Input: part model. Units: mm. Frame: model coordinates. A direction names the side the tool comes from. Give positions to 0.01 mm unless a question says otherwise; leave off trailing zeros. Loops run counter-clockwise (first coordinate to the right, second up) from the corner with the lowest first, then second, coordinate; pieces in that order, holes last. Notation, with made-up numbers: (-15.75, -33.75) - (37.25, -33.75) arc R10 cw to (37.25, -29.75) - close; hole circle Ø6 at (66.5, -18). An arc over 180 degrees is marked (long way). One line per item, written item: value.
from build123d import *

# Parameters (mm, degrees)
BOSS_EXTRUDE1_DEPTH     = 32
SKETCH2_R               = 22.5
BOSS_EXTRUDE4_DEPTH     = 10
CUT_EXTRUDE1_DEPTH      = 80.029560932
CUT_EXTRUDE1_DEPTH_BACK = 80.029560932
SKETCH3_R               = 5
FILLET3_R               = 11
FILLET4_RADIUS          = 16
FILLET4_LENGTH          = 4.5
FILLET5_RADIUS          = 16
FILLET5_LENGTH          = 4.5
CUT_EXTRUDE2_DEPTH      = 74.711106836
CUT_EXTRUDE2_DEPTH_BACK = 74.711106836
SKETCH4_R               = 3


with BuildPart() as part:
    # Sketch1 → Boss-Extrude1 (new body)
    with BuildSketch(Plane.XY):
        Polygon((-19.112903226, 28.185483871), (-19.112903226, -26.814516129), (43.887096774, -26.814516129), (43.887096774, 28.185483871), (39.387096774, 28.185483871), (39.387096774, -16.814516129), (-14.612903226, -16.814516129), (-14.612903226, 28.185483871), align=None)
    extrude(amount=BOSS_EXTRUDE1_DEPTH)

    # Sketch2 → Boss-Extrude4 (add)
    with BuildSketch(Plane.XZ.offset(26.814516129)):
        with Locations((12.887096774, 16)):
            Circle(SKETCH2_R)
    extrude(amount=-BOSS_EXTRUDE4_DEPTH)

    # Sketch3 → Cut-Extrude1 (cut, two sides: drawn at the far end of the back side and taken through both)
    with BuildSketch(Plane(origin=(43.887096774, 0, 0), x_dir=(0, 0, -1), z_dir=(1, 0, 0)).offset(-CUT_EXTRUDE1_DEPTH_BACK)):
        with Locations(Location((-16, 12.185483871, 0), (0, 0, 90))):
            Circle(SKETCH3_R)
    extrude(amount=CUT_EXTRUDE1_DEPTH + CUT_EXTRUDE1_DEPTH_BACK, mode=Mode.SUBTRACT)

    # Fillet3
    fillet3_edges = [part.edges().sort_by_distance(p)[0] for p in [
        (-14.612903226, -16.814516129, 16),
        (39.387096774, -16.814516129, 16),
        (43.887096774, -26.814516129, 16),
        (-19.112903226, -26.814516129, 16),
    ]]
    fillet(fillet3_edges, radius=FILLET3_R)

    # Fillet4: full round fillet: the end face becomes a half cylinder, R = half its width
    fillet4_face = Plane((41.637096774, 28.185483871, 16), x_dir=(1, 0, 0), z_dir=(0, 1, 0))  # on the end face: x along it, z out of the body
    fillet4_slab = fillet4_face.offset(-FILLET4_RADIUS / 2) * Box(FILLET4_LENGTH, 2 * FILLET4_RADIUS, FILLET4_RADIUS, mode=Mode.PRIVATE)  # the body's end, R deep
    fillet4_round = Plane((41.637096774, 12.185483871, 16), x_dir=(0, 1, 0), z_dir=(1, 0, 0)) * Cylinder(FILLET4_RADIUS, FILLET4_LENGTH, mode=Mode.PRIVATE)  # its axis R under the face
    add(fillet4_slab - fillet4_round, mode=Mode.SUBTRACT)

    # Fillet5: full round fillet: the end face becomes a half cylinder, R = half its width
    fillet5_face = Plane((-16.862903226, 28.185483871, 16), x_dir=(-1, 0, 0), z_dir=(0, 1, 0))  # on the end face: x along it, z out of the body
    fillet5_slab = fillet5_face.offset(-FILLET5_RADIUS / 2) * Box(FILLET5_LENGTH, 2 * FILLET5_RADIUS, FILLET5_RADIUS, mode=Mode.PRIVATE)  # the body's end, R deep
    fillet5_round = Plane((-16.862903226, 12.185483871, 16), x_dir=(0, 1, 0), z_dir=(-1, 0, 0)) * Cylinder(FILLET5_RADIUS, FILLET5_LENGTH, mode=Mode.PRIVATE)  # its axis R under the face
    add(fillet5_slab - fillet5_round, mode=Mode.SUBTRACT)

    # Sketch4 → Cut-Extrude2 (cut, two sides: drawn at the far end of the back side and taken through both)
    with BuildSketch(Plane(origin=(0, -16.814516129, 0), x_dir=(1, 0, 0), z_dir=(0, 1, 0)).offset(-CUT_EXTRUDE2_DEPTH_BACK)):
        with Locations(Location((12.387096774, -4.010421192, 0), (0, 0, 180))):
            Circle(SKETCH4_R)
        with Locations(Location((24.876675582, -15.5, 0), (0, 0, 180))):
            Circle(SKETCH4_R)
        with Locations(Location((13.387096774, -27.989578808, 0), (0, 0, 180))):
            Circle(SKETCH4_R)
        with Locations(Location((0.897517966, -16.5, 0), (0, 0, 180))):
            Circle(SKETCH4_R)
    extrude(amount=CUT_EXTRUDE2_DEPTH + CUT_EXTRUDE2_DEPTH_BACK, mode=Mode.SUBTRACT)


solid = part.part
Item 1: Draft query along Z for faces 5 (the face through (-11.305, -13.678, 16.224)), 6 (the face through (-15, -11, 0)), 7 (the face through (41.61, 11.1, 11.12)). Return one class per face: pulls with the +Z half, pulls with the -Z half, needs draft (parallel to the pull), parting line crosses it, or undercut.
Verdict:
face 5: needs draft
face 6: pulls with the -Z half
face 7: undercut
Item 2: Section B-B, the plane x = -10. Output: boundary loops of the cut face in (y, z).
Verdict:
outline: (-26.65, 0) - (-14.77, 0) - (-14.77, 32) - (-26.65, 32) - close
Item 3: Pin query (flat end, axial travel): P1, Ø16, axis at y = 12.19, z = 16, coming from the +X side; P2, Ø4.5, axis at x = 36, y = -7.5, coming from the -Z side; P3, Ø7.5, axis at x = 38, y = -3.5, coming from the +Z side; P4, Ø8, axis at x = -10, y = -13.5, coming from the -Z side. Return the tip coordinate at first contact, or that it passes through.
Verdict:
P1: stops at x = 43.89
P2: passes through
P3: stops at z = 32
P4: stops at z = 0
Item 4: Material intervals for L1, parallel to X at y = 15, z = 30.5; L2, parallel to Y at x = 29, z = 23; L3, parallel to X at y = -7.5, z = 17.5, sorted ascending.
Verdict:
L1: x = -19.11 to -14.61, 39.39 to 43.89
L2: y = -26.81 to -16.8
L3: x = -19.11 to -14.48, 39.26 to 43.89
Item 5: Section A-A, the plane y = 1. Output: boundary loops of the cut face in (x, z).
Verdict:
outline: (-19.11, 0) - (-14.61, 0) - (-14.61, 32) - (-19.11, 32) - close; (39.39, 0) - (43.89, 0) - (43.89, 32) - (39.39, 32) - close
Item 6: Access query for faces 1 (the face through (-15, -11, 32)), 2 (the face through (40, -11, 32)), 3 (the face through (40, -11, 0)), 4 (the face through (-14.613, 7, 16)). Directions: +Z, -Z, +X, -X, +Y, -Y. A direction counts if a zero-diameter tool reaches every point of the face in a straight line with its end or side. Return the directions, or none.
Verdict:
face 1: +Z, -X, +Y, -Y
face 2: +Z, +X, +Y, -Y
face 3: -Z, +X, +Y, -Y
face 4: +Z, -Z, +Y
Item 7: Section C-C, the plane z = -3. Output: boundary loops of the cut face in (x, y), and give its area (3 significant figures).
Verdict:
outline: (0.84, -26.81) - (24.94, -26.81) - (24.94, -16.81) - (0.84, -16.81) - close
area: 241 mm^2
